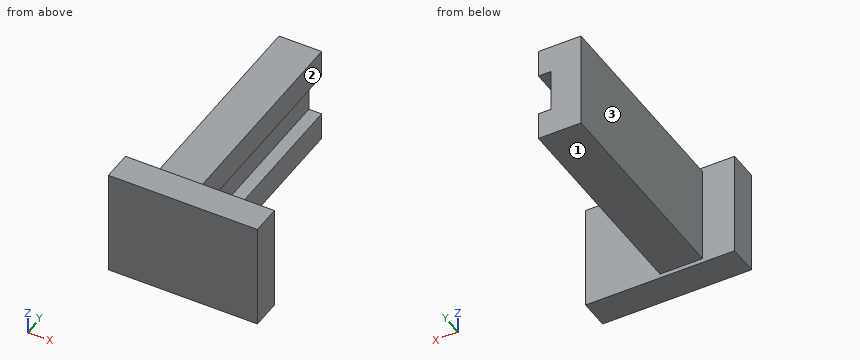
from build123d import *

# Parameters (mm, degrees)
CROQUIS1_W              = 175
CROQUIS1_H              = 125
SALIENTE_EXTRUIR1_DEPTH = 35
CROQUIS2_W              = 50
CROQUIS2_H              = 115
SALIENTE_EXTRUIR2_DEPTH = 250
CROQUIS3_W              = 50
CROQUIS3_H              = 250
CORTAR_EXTRUIR1_DEPTH   = 15


with BuildPart() as part:
    # Croquis1 → Saliente-Extruir1 (new body)
    with BuildSketch(Plane(origin=(0, 0, 0), x_dir=(1, 0, 0), z_dir=(0, 1, 0))):
        Rectangle(CROQUIS1_W, CROQUIS1_H)
    extrude(amount=SALIENTE_EXTRUIR1_DEPTH)

    # Croquis2 → Saliente-Extruir2 (add)
    with BuildSketch(Plane(origin=(0, 35, 0), x_dir=(1, 0, 0), z_dir=(0, 1, 0))):
        with Locations((-25, 0)):
            Rectangle(CROQUIS2_W, CROQUIS2_H)
    extrude(amount=SALIENTE_EXTRUIR2_DEPTH)

    # Croquis3 → Cortar-Extruir1 (cut)
    with BuildSketch(Plane(origin=(0, 0, 0), x_dir=(0, 0, -1), z_dir=(1, 0, 0))):
        with Locations((0, 160)):
            Rectangle(CROQUIS3_W, CROQUIS3_H)
    extrude(amount=-CORTAR_EXTRUIR1_DEPTH, mode=Mode.SUBTRACT)


solid = part.part
Verification items for the finished model (mm, model axes). Face numbers are marked on the shaded views. A direction names the side the tool comes from. Give positions to 0.01 mm unless a question says otherwise; leave off trailing zeros. Loops run counter-clockwise (first coordinate to the right, second up) from the corner with the lowest first, then second, coordinate; pieces in that order, holes last.
1) Sectioned sample at A-A, the plane y = 259. Enter the section's corners in (x, z), then the cut area to 3 significant figures.
2) Set-up check for the marked faces 1, 2 and 3: record each of +Z, -Z, +X, -X, +Y, -Y from which the full face is reachable in a straight line by a thin tool's end or side.
3) Depth check by flat-ended pin: pin 1 Ø3 at (x, z) = (12.5, -22) entering from +Y; pin 2 Ø7.5 at (x, y) = (-8, 152.5) entering from +Z; pin 3 Ø12 at (x, y) = (-10, 220.5) entering from -Z. Enter the tip coordinate at first touch or a pass-through.
4) Sectioned sample at B-B, the plane z = 41. Enter the section's corners in (x, y).
5) Sectioned sample at C-C, the plane x = 66. Enter the section's corners in (y, z), then the cut area to 4 significant figures.
6) Thickness scan on line 1 along Z through (x, y) = (-9.5, 125.5); line 2 along Y through (x, z) = (2.5, 52); line 3 along X through (y, z) = (205.5, 32.5). Record the ranges inside material, lowest first.
Answers:
1. outline: (-50, -57.5) - (0, -57.5) - (0, -25) - (-15, -25) - (-15, 25) - (0, 25) - (0, 57.5) - (-50, 57.5) - close
1. area: 5,000 mm2
2. face 1: -Z, +X, -X, +Y
2. face 2: +Z, -Z, +X, +Y
2. face 3: +Z, -Z, -X, +Y
3. pin 1: stops at y = 35
3. pin 2: stops at z = 57.5
3. pin 3: stops at z = -57.5
4. outline: (-87.5, 0) - (87.5, 0) - (87.5, 35) - (0, 35) - (0, 285) - (-50, 285) - (-50, 35) - (-87.5, 35) - close
5. outline: (0, -62.5) - (35, -62.5) - (35, 62.5) - (0, 62.5) - close
5. area: 4,375 mm2
6. line 1: z = -57.5 to -25, 25 to 57.5
6. line 2: y = 0 to 35
6. line 3: x = -50 to 0
